```python
from build123d import *

# Parameters (mm, degrees)
F1_W     = 100
F1_H     = 100
F2_DEPTH = 25
F3_R     = 25
F4_R     = 5
F5_W     = 25
F5_H     = 20
F6_DEPTH = 10
F6_TAPER = 3
F7_R     = 5
F8_R     = 22.5
F9_DEPTH = 10


with BuildPart() as f2:
    # F1 (on Top) → F2 (new body)
    with BuildSketch(Plane.XY):
        Rectangle(F1_W, F1_H)
    extrude(amount=F2_DEPTH)

    # F3
    f3_edges = [f2.edges().sort_by_distance(p)[0] for p in [
        (50, -50, 12.5),
        (-50, -50, 12.5),
        (-50, 50, 12.5),
        (50, 50, 12.5),
    ]]
    fillet(f3_edges, radius=F3_R)

    # F4
    f4_edges = [f2.edges().sort_by_distance(p)[0] for p in [
        (0, -50, 25),
        (-42.67767, -42.67767, 25),
        (42.67767, -42.67767, 25),
        (-50, 0, 25),
        (50, 0, 25),
        (-42.67767, 42.67767, 25),
        (42.67767, 42.67767, 25),
        (0, 50, 25),
        (0, -50, 0),
        (-42.67767, -42.67767, 0),
        (42.67767, -42.67767, 0),
        (-50, 0, 0),
        (50, 0, 0),
        (-42.67767, 42.67767, 0),
        (42.67767, 42.67767, 0),
        (0, 50, 0),
    ]]
    fillet(f4_edges, radius=F4_R)

    # F5 (on face) → F6 (join)
    with BuildSketch(Plane.XY.offset(25)):
        Rectangle(F5_W, F5_H)
    extrude(amount=F6_DEPTH, taper=F6_TAPER)

    # F7
    f7_edges = [f2.edges().sort_by_distance(p)[0] for p in [
        (0, -45, 25),
        (-39.142136, -39.142136, 25),
        (39.142136, -39.142136, 25),
        (-45, 0, 25),
        (45, 0, 25),
        (-39.142136, 39.142136, 25),
        (39.142136, 39.142136, 25),
        (0, 45, 25),
        (12.5, 0, 25),
        (0, 10, 25),
        (-12.5, 0, 25),
        (0, -10, 25),
    ]]
    fillet(f7_edges, radius=F7_R)

    # F8 (on face) → F9 (cut)
    with BuildSketch(Plane(origin=(0, 0, 0), x_dir=(1, 0, 0), z_dir=(0, 0, -1))):
        Circle(F8_R)
    extrude(amount=-F9_DEPTH, mode=Mode.SUBTRACT)


solid = f2.part
```
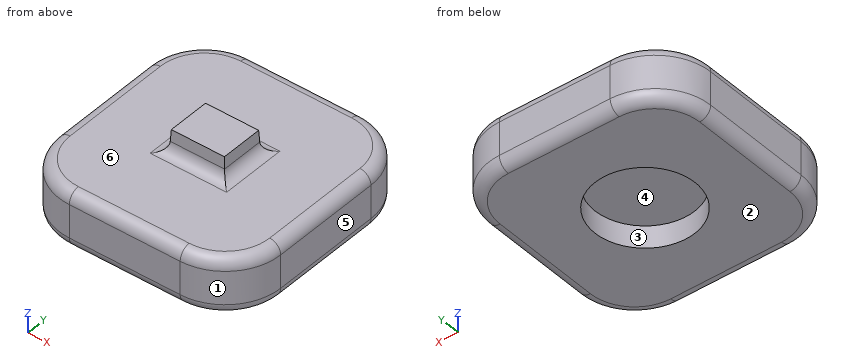
Model file for the job. Use its own axes, mm. Face numbers are marked on the shaded views. A direction names the side the tool comes from. Coordinates: 2 decimals unless noted, no trailing zeros. Loops run counter-clockwise (first coordinate to the right, second up) from the corner with the lowest first, then second, coordinate; pieces in that order, holes last. Notation, with made-up numbers: (-34, 40) -> (-6, 40) arc R24 cw to (-6, 71) -> close; hole circle Ø6 at (38, 24.25). An arc over 180 degrees is marked (long way). Answer as a JSON object with one key per item and string values.
Q1. 3-axis set-ups, long thin cutter, end or side, ignore diameter. For the marked faces 4, 5 and 6: which of +Z, -Z, +X, -X, +Y, -Y reach the whole face in a straight line?
Report:
{"face 4": "-Z", "face 5": "+Z, -Z, +X, +Y, -Y", "face 6": "+Z"}
Q2. Probe probe 1 along X at (y, z) = (0, 5); probe 2 along Z at (x, y) = (11.5, -19.5). List the from-to ranges inside material, lowest first.
Report:
{"probe 1": "x = -50 to -22.5, 22.5 to 50", "probe 2": "z = 0 to 25"}
Q3. Cut at A-A (y = 0). List the corners of the cut face in (x, z), and give its area (3 significant figures).
Report:
{"outline": "(-50, 5) arc R5 ccw to (-45, 0) -> (-22.5, 0) -> (-22.5, 10) -> (22.5, 10) -> (22.5, 0) -> (45, 0) arc R5 ccw to (50, 5) -> (50, 20) arc R5 ccw to (45, 25) -> (17.24, 25) arc R5 cw to (12.25, 29.74) -> (11.98, 35) -> (-11.98, 35) -> (-12.25, 29.74) arc R5 cw to (-17.24, 25) -> (-45, 25) arc R5 ccw to (-50, 20) -> close", "area": "2,280 mm2"}
Q4. Cut at C-C (z = 7). List the corners of the cut face in (x, y), and give its area (3 significant figures).
Report:
{"outline": "(-50, -25) arc R25 ccw to (-25, -50) -> (25, -50) arc R25 ccw to (50, -25) -> (50, 25) arc R25 ccw to (25, 50) -> (-25, 50) arc R25 ccw to (-50, 25) -> close; hole circle Ø45 at (0, 0)", "area": "7,870 mm2"}
Q5. Flat gauge pins, fed straight in: P1, Ø6, axis at x = -2.5, z = 4.5, coming from the +Y side; P2, Ø6, axis at x = 19.5, y = 26.5, coming from the +Z side; P3, Ø6, axis at x = 15.5, y = 16.5, coming from the +Z side. Where does each tip first touch, or does it go through?
Report:
{"P1": "stops at y = 50", "P2": "stops at z = 25", "P3": "stops at z = 25.16"}
Q6. Cut at D-D (z = 32.5). List the corners of the cut face in (x, y).
Report:
{"outline": "(-12.11, -9.61) -> (12.11, -9.61) -> (12.11, 9.61) -> (-12.11, 9.61) -> close"}
Q7. Pull direction X, two halves, no side cores. Call the marked faces 1, 2 and 3: released by +X, released by -X, zero draft, split by the parting line, or undercut.
Report:
{"face 1": "released by +X", "face 2": "zero draft", "face 3": "undercut"}
Q8. Cut at B-B (x = 0). List the corners of the cut face in (y, z), and give its area (3 significant figures).
Report:
{"outline": "(-50, 5) arc R5 ccw to (-45, 0) -> (-22.5, 0) -> (-22.5, 10) -> (22.5, 10) -> (22.5, 0) -> (45, 0) arc R5 ccw to (50, 5) -> (50, 20) arc R5 ccw to (45, 25) -> (14.74, 25) arc R5 cw to (9.75, 29.74) -> (9.48, 35) -> (-9.48, 35) -> (-9.75, 29.74) arc R5 cw to (-14.74, 25) -> (-45, 25) arc R5 ccw to (-50, 20) -> close", "area": "2,230 mm2"}
